```python
from build123d import *

# Parameters (mm, degrees)
F0_W      = 109.6809846
F0_H      = 62.036204
F0_R      = 2.15265
F0_W_2    = 9.525
F0_H_2    = 6
F0_R_2    = 11.1125
F1_DEPTH  = 19.05
F2_W      = 9.525
F2_H      = 9.525
F3_DEPTH  = 12.7
F4_R      = 4.76249
F6_DEPTH  = 19.05
F7_R      = 2.15265
F8_DEPTH  = 3.175
F9_R      = 1.7272
F10_DEPTH = 3.525


# Not quite as in the source:
# - a fillet or chamfer is up to 0.001 mm smaller than in the source, because OpenCascade refuses the exact size


with BuildPart() as f1:
    # F0 (on Top) → F1 (new body)
    with BuildSketch(Plane.XY):
        with Locations((0, -16.730602)):
            Rectangle(F0_W, F0_H)
        with Locations((-50.0779923, -42.986204)):
            Circle(F0_R, mode=Mode.SUBTRACT)
        with Locations((27.406219, -41.573704)):
            Rectangle(F0_W_2, F0_H_2, mode=Mode.SUBTRACT)
        with Locations((50.0779923, -42.986204)):
            Circle(F0_R, mode=Mode.SUBTRACT)
        with Locations((-40.5529923, 0)):
            Circle(F0_R_2, mode=Mode.SUBTRACT)
        with Locations((-21.5029923, 9.525)):
            Circle(F0_R, mode=Mode.SUBTRACT)
        with Locations((21.5029923, 9.525)):
            Circle(F0_R, mode=Mode.SUBTRACT)
        with Locations((40.5529923, 0)):
            Circle(F0_R_2, mode=Mode.SUBTRACT)
    extrude(amount=F1_DEPTH)

    # F2 (on face) → F3 (cut)
    with BuildSketch(Plane.XY.offset(19.05)):
        with Locations((-21.5029923, 9.525)):
            Rectangle(F2_W, F2_H)
        with Locations((21.5029923, 9.525)):
            Rectangle(F2_W, F2_H)
        with Locations((50.0779923, -42.986204)):
            Rectangle(F2_W, F2_H)
        with Locations((-50.0779923, -42.986204)):
            Rectangle(F2_W, F2_H)
    extrude(amount=-F3_DEPTH, mode=Mode.SUBTRACT)

    # F4 (radius 4.7625 in the source; OpenCascade refuses exactly that, so slightly less here)
    f4_edges = [f1.edges().sort_by_distance(p)[0] for p in [
        (-45.315492, -38.223704, 12.7),
        (45.315492, -38.223704, 12.7),
        (16.740492, 4.7625, 12.7),
        (26.265492, 4.7625, 12.7),
        (-16.740492, 4.7625, 12.7),
        (-26.265492, 4.7625, 12.7),
    ]]
    fillet(f4_edges, radius=F4_R)

    # F5 (on face) → F6 (cut, through all)
    with BuildSketch(Plane.XY.offset(19.05)):
        with BuildLine():
            Line((-51.6654923, -23.080602), (-1.5875, -23.080602))
            Line((-1.5875, -23.080602), (-1.5875, 11.1125))
            Line((-1.5875, 11.1125), (-13.5654923, 11.1125))
            Line((-13.5654923, 11.1125), (-13.5654923, 9.525))
            ThreePointArc((-13.5654923, 9.525), (-15.8903322243, 3.9123399243), (-21.5029923, 1.5875))
            Line((-21.5029923, 1.5875), (-26.2654923, 1.5875))
            Line((-26.2654923, 1.5875), (-26.2654923, 0))
            ThreePointArc((-26.2654923, 0), (-30.4502041638, -10.1027881362), (-40.5529923, -14.2875))
            Line((-40.5529923, -14.2875), (-51.6654923, -14.2875))
            Line((-51.6654923, -14.2875), (-51.6654923, -23.080602))
        make_face()
        with BuildLine():
            Line((-1.5875, -44.573704), (-1.5875, -26.255602))
            Line((-1.5875, -26.255602), (-51.6654923, -26.255602))
            Line((-51.6654923, -26.255602), (-51.6654923, -35.048704))
            Line((-51.6654923, -35.048704), (-50.0779923, -35.048704))
            ThreePointArc((-50.0779923, -35.048704), (-44.4653322243, -37.3735439243), (-42.1404923, -42.986204))
            Line((-42.1404923, -42.986204), (-42.1404923, -44.573704))
            Line((-42.1404923, -44.573704), (-1.5875, -44.573704))
        make_face()
        with BuildLine():
            Line((1.5875, -23.080602), (51.6654923, -23.080602))
            Line((51.6654923, -23.080602), (51.6654923, -14.2875))
            Line((51.6654923, -14.2875), (40.5529923, -14.2875))
            ThreePointArc((40.5529923, -14.2875), (30.4502041638, -10.1027881362), (26.2654923, 0))
            Line((26.2654923, 0), (26.2654923, 1.5875))
            Line((26.2654923, 1.5875), (21.5029923, 1.5875))
            ThreePointArc((21.5029923, 1.5875), (15.8903322243, 3.9123399243), (13.5654923, 9.525))
            Line((13.5654923, 9.525), (13.5654923, 11.1125))
            Line((13.5654923, 11.1125), (1.5875, 11.1125))
            Line((1.5875, 11.1125), (1.5875, -23.080602))
        make_face()
        with BuildLine():
            Line((51.6654923, -26.255602), (1.5875, -26.255602))
            Line((1.5875, -26.255602), (1.5875, -44.573704))
            Line((1.5875, -44.573704), (19.468719, -44.573704))
            Line((19.468719, -44.573704), (19.468719, -35.048704))
            Line((19.468719, -35.048704), (35.343719, -35.048704))
            Line((35.343719, -35.048704), (35.343719, -44.573704))
            Line((35.343719, -44.573704), (42.1404923, -44.573704))
            Line((42.1404923, -44.573704), (42.1404923, -42.986204))
            ThreePointArc((42.1404923, -42.986204), (44.4653322243, -37.3735439243), (50.0779923, -35.048704))
            Line((50.0779923, -35.048704), (51.6654923, -35.048704))
            Line((51.6654923, -35.048704), (51.6654923, -26.255602))
        make_face()
    extrude(amount=-F6_DEPTH, mode=Mode.SUBTRACT)

    # F7 (on face) → F8 (cut, through all)
    with BuildSketch(Plane.XZ.offset(47.748704)):
        with Locations((27.406219, 9.525)):
            Circle(F7_R)
    extrude(amount=-F8_DEPTH, mode=Mode.SUBTRACT)

    # F9 (on face) → F10 (cut, through all)
    with BuildSketch(Plane.XZ.offset(38.573704)):
        with Locations((27.406219, 9.525)):
            Circle(F9_R)
    extrude(amount=-F10_DEPTH, mode=Mode.SUBTRACT)


solid = f1.part
```
Geometry: final body of the model. Coordinates: model frame, mm. A direction names the side the tool comes from. Give positions to 0.01 mm unless a question says otherwise; leave off trailing zeros. Write each loop counter-clockwise with the first axis right and the second up, starting at its lowest first coordinate (ties: lowest second). Pieces come first, ordered by that corner, then holes.
1. Draft query along Y for faces 1 (the cylindrical face through (46.75, -39.58, 12.61)), 2 (the flat face through (-7, 11.112, 10)), 3 (the flat face through (-26.265, 12, 13)). Return one class per face: released by +Y, released by -Y, zero draft, split by the parting line, or undercut.
2. Line query: probe 1 along X at (y, z) = (-44, 10.75); probe 2 along Y at (x, z) = (-2, 2.75); probe 3 along X at (y, z) = (12, 12). Output: solid intervals per line, ascending.
3. Section query C-C, the plane z = 5. Count the separate pieces of the cut face and the enclosed holes in it, then the cut area to 3 significant figures.
4. Pin query (flat end, axial travel): P1, Ø2.5, axis at x = 53, z = 13, coming from the -Y side. Return the tip coordinate at first contact, or that it passes through.
5. Section query A-A, the plane x = 12.5. Return loops of the section in (y, z), then the cut area to 3 significant figures.
6. Reachability of faces 4 (the flat face through (32.169, -42, 9)), 5 (the flat face through (-16.74, 12, 13)), 6 (the flat face through (52, -38.224, 13)), 7 (the cylindrical face through (25.82, -46.18, 10.98)) from +Z, -Z, +X, -X, +Y, -Y: full face, straight path, thin tool, end or side. Return the list, or none.
7. Section query B-B, the plane y = -27.5. Return loops of the section in (x, z).
Computed:
1. face 1: released by -Y
1. face 2: undercut
1. face 3: zero draft
2. probe 1: x = -45.32 to -42.14, -1.59 to 1.59, 19.47 to 22.64, 32.17 to 35.34, 42.14 to 45.32
2. probe 2: y = -47.75 to -44.57, -26.26 to -23.08, 11.11 to 14.29
2. probe 3: x = -54.84 to -26.27, -16.74 to 16.74, 26.27 to 54.84
3. separate pieces: 1
3. enclosed holes: 11
3. area: 2,380 mm2
4. P1: stops at y = -38.22
5. outline: (-47.75, 0) - (-44.57, 0) - (-44.57, 19.05) - (-47.75, 19.05) - close; (-26.26, 0) - (-23.08, 0) - (-23.08, 19.05) - (-26.26, 19.05) - close; (11.11, 0) - (14.29, 0) - (14.29, 19.05) - (11.11, 19.05) - close
5. area: 181 mm2
6. face 4: +Z, -Z
6. face 5: +Z, +Y
6. face 6: +Z, +X, -Y
6. face 7: -Y
7. outline: (-54.84, 0) - (-51.67, 0) - (-51.67, 19.05) - (-54.84, 19.05) - close; (-1.59, 0) - (1.59, 0) - (1.59, 19.05) - (-1.59, 19.05) - close; (51.67, 0) - (54.84, 0) - (54.84, 19.05) - (51.67, 19.05) - close
